```python
from build123d import *

# Parameters (mm, degrees)
BODY_DEPTH     = 5.5626
THREAD_D       = 4.9784
CHAMFER2_SIZE  = 0.687407664
CHAMFER2_SIZE2 = 0.396875
CHAMFER3_SIZE  = 0.687407664
CHAMFER3_SIZE2 = 0.396875


with BuildPart() as part:
    # Sketch1 → Body (new body)
    with BuildSketch(Plane.YZ):
        Polygon((-6.415804866, 0), (-3.207902433, 5.55625), (3.207902433, 5.55625), (6.415804866, 0), (3.207902433, -5.55625), (-3.207902433, -5.55625), align=None)
    extrude(amount=BODY_DEPTH)

    # Sketch2 → Chamfer1 (revolve, cut)
    with BuildSketch(Plane.XY):
        Polygon((0, 5.55625), (0.496264233, 6.415804866), (0, 6.415804866), align=None)
        Polygon((5.5626, 5.55625), (5.5626, 6.415804866), (5.066335767, 6.415804866), align=None)
    revolve(axis=Axis((-1.11252, 0, 0), (1, 0, 0)), mode=Mode.SUBTRACT)

    # Thread (through all)
    with Locations(Plane(origin=(5.5626, 0, 0), x_dir=(0, 0, -1), z_dir=(1, 0, 0))):
        with Locations((0, 0)):
            Hole(THREAD_D / 2)

    # Chamfer2
    chamfer2_edges = [part.edges().sort_by_distance(p)[0] for p in [
        (5.5626, 0, -2.4892),
    ]]
    chamfer2_side = [part.faces().sort_by_distance(p)[0] for p in [
        (5.5626, -5.399095518, -9.9e-08),
    ]]
    chamfer(chamfer2_edges, length=CHAMFER2_SIZE, length2=CHAMFER2_SIZE2, reference=chamfer2_side[0])

    # Chamfer3
    chamfer3_edges = [part.edges().sort_by_distance(p)[0] for p in [
        (0, 0, -2.4892),
    ]]
    chamfer3_side = [part.faces().sort_by_distance(p)[0] for p in [
        (0, -5.399095518, -9.9e-08),
    ]]
    chamfer(chamfer3_edges, length=CHAMFER3_SIZE, length2=CHAMFER3_SIZE2, reference=chamfer3_side[0])


solid = part.part
```
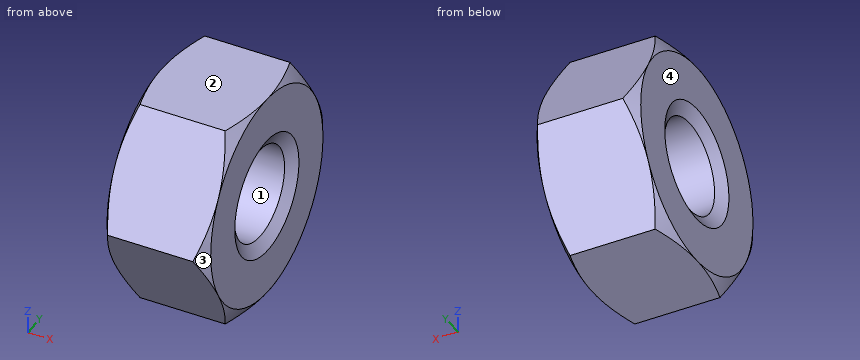
For this review, take the finished solid that the model builds, in its own axes (mm). Face numbers are marked on the shaded views. Coordinates: 2 decimals unless noted, no trailing zeros. Write each loop counter-clockwise with the first axis right and the second up, starting at its lowest first coordinate (ties: lowest second). Pieces come first, ordered by that corner, then holes.
(1) For pin 1 Ø1 at (y, z) = (-0.5, 2) entering from +X, flat-tipped, find the tip position at first contact; note if it passes through.
(2) Add section A-A on x = 2.9. Give the boundary of the cut face in (y, z), then the cut area to 3 significant figures.
(3) The part is to be moulded in two halves that separate along Z. For the marked faces 1, 2, 3 and 4, say which applies: +Z half, -Z half, draft (parallel to the pull), parting line (faces both ways), or undercut.
(4) Wall thickness on probe 1 along Y at (x, z) = (1.5, -0.25); probe 2 along Z at (x, y) = (4.5, -2.25); probe 3 along Z at (x, y) = (1, -0.5): over which ranges is each line inside the solid? List them lowest first.
Answer sheet:
1. pin 1: stops at x = 5.21
2. outline: (-6.42, 0) - (-3.21, -5.56) - (3.21, -5.56) - (6.42, 0) - (3.21, 5.56) - (-3.21, 5.56) - close; hole circle Ø4.98 at (0, 0)
2. area: 87.5 mm2
3. face 1: undercut
3. face 2: +Z half
3. face 3: parting line
3. face 4: draft
4. probe 1: y = -6.27 to -2.48, 2.48 to 6.27
4. probe 2: z = -5.56 to -1.06, 1.06 to 5.56
4. probe 3: z = -5.56 to -2.44, 2.44 to 5.56
